```python
from build123d import *

# Parameters (mm, degrees)
F0_W     = 42
F0_H     = 82
F1_DEPTH = 3
F2_W     = 42
F2_H     = 82
F2_W_2   = 35
F2_H_2   = 76
F3_DEPTH = 18
F4_W     = 12
F4_H     = 82
F5_DEPTH = 3
F7_DEPTH = 25
F8_DEPTH = 25
F9_R     = 3
F10_R    = 5


with BuildPart() as f1:
    # F0 (on Top) → F1 (new body)
    with BuildSketch(Plane.XY):
        Rectangle(F0_W, F0_H)
    extrude(amount=F1_DEPTH)

    # F2 (on face) → F3 (join)
    with BuildSketch(Plane.XY.offset(3)):
        Rectangle(F2_W, F2_H)
        Rectangle(F2_W_2, F2_H_2, mode=Mode.SUBTRACT)
    extrude(amount=F3_DEPTH)

    # F4 (on face) → F5 (join)
    with BuildSketch(Plane.XY.offset(21)):
        with Locations((-23.5, 0)):
            Rectangle(F4_W, F4_H)
        with Locations((23.5, 0)):
            Rectangle(F4_W, F4_H)
    extrude(amount=F5_DEPTH)

    # F6 (on face) → F7 (cut)
    with BuildSketch(Plane(origin=(0, 0, 0), x_dir=(1, 0, 0), z_dir=(0, 0, -1))):
        Polygon((13, 7.8317355365), (13, 33), (3.5048450809, 33), (-13, 33), (-13, 14.662142843), (-13, -41), (13, -41), align=None)
    extrude(amount=-F7_DEPTH, mode=Mode.SUBTRACT)

    # F8 (cut): faces of the model
    f8_faces = [f1.faces().sort_by_distance(p)[0] for p in [
        (15.25, 38, 12),
        (-15.25, 38, 12),
    ]]
    extrude(f8_faces, amount=-F8_DEPTH, mode=Mode.SUBTRACT)

    # F9
    f9_edges = [f1.edges().sort_by_distance(p)[0] for p in [
        (-21, 0, 0),
        (0, -41, 0),
        (21, 0, 0),
        (-13, 41, 1.5),
        (13, 41, 1.5),
    ]]
    fillet(f9_edges, radius=F9_R)

    # F10
    f10_edges = [f1.edges().sort_by_distance(p)[0] for p in [
        (29.5, -41, 22.5),
        (-29.5, -41, 22.5),
        (-29.5, 41, 22.5),
        (29.5, 41, 22.5),
    ]]
    fillet(f10_edges, radius=F10_R)


solid = f1.part
```
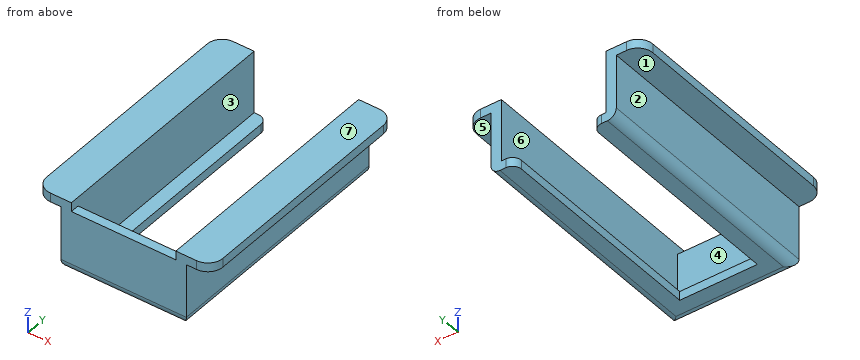
Check sheet for the modelled part. Datum: model origin and axes. Units: mm. Face numbers are marked on the shaded views. A direction names the side the tool comes from. Give positions to 0.01 mm unless a question says otherwise; leave off trailing zeros. Order: outer loops, then holes, each group sorted by start corner. A loop starts at its lowest first (then second) coordinate and runs counter-clockwise, first axis right, second up. Notation, with made-up numbers: (47, 32) -> (79, 32) arc R12 cw to (79, 55) -> close; hole circle Ø1 at (-15, 81.5). An arc over 180 degrees is marked (long way). Use CSV: the item, a comma, the result in double quotes. Start each with the question number.
1) Set-up check for the marked faces 5, 6 and 7: record each of +Z, -Z, +X, -X, +Y, -Y from which the full face is reachable in a straight line by a thin tool's end or side.
2) Mould release check, pull along X, two halves, no side actions. Record for the marked faces 1, 2, 3 and 4: released by +X, released by -X, zero draft, split by the parting line, or undercut.
3) Sectioned sample at D-D, the plane z = 5. Record the boundary of the cut face in (x, y), plus the area to 3 significant figures.
4) Sectioned sample at B-B, the plane x = 3. Record the boundary of the cut face in (y, z).
5) Sectioned sample at A-A, the plane z = 22.75. Record the boundary of the cut face in (x, y).
6) Sectioned sample at C-C, the plane y = -12.5. Record the boundary of the cut face in (x, z).
7) Material ranges on line 1 (X direction, y = 21.5, z = 14.75); line 2 (X direction, y = 2, z = 2.75); line 3 (Z direction, x = 22, y = 35), recorded low to high. Write a range as from..to.
8) Go/stop test with flat-tipped pins: P1, Ø2.5, axis at x = -1.5, z = 1.5, coming from the +Y side; P2, Ø2.5, axis at y = -5, z = 1, coming from the +X side; P3, Ø1.5, axis at x = -6.5, z = 16.5, coming from the +Y side. Record where each tip stops, or that it passes through.
Recorded:
1,face 5,"-Z, +X, +Y, -Y"
1,face 6,"+Z, +Y"
1,face 7,"+Z, +X, -X, +Y, -Y"
2,face 1,"zero draft"
2,face 2,"released by -X"
2,face 3,"undercut"
2,face 4,"undercut"
3,outline,"(-21, -41) -> (21, -41) -> (21, 41) -> (17.5, 41) -> (17.5, -38) -> (-17.5, -38) -> (-17.5, 41) -> (-21, 41) -> close"
3,area,"679 mm2"
4,outline,"(-41, 3) arc R3 ccw to (-38, 0) -> (-33, 0) -> (-33, 3) -> (-38, 3) -> (-38, 21) -> (-41, 21) -> close"
5,outline,"(-29.5, -36) arc R5 ccw to (-24.5, -41) -> (-17.5, -41) -> (-17.5, 41) -> (-24.5, 41) arc R5 ccw to (-29.5, 36) -> close; (17.5, -41) -> (24.5, -41) arc R5 ccw to (29.5, -36) -> (29.5, 36) arc R5 ccw to (24.5, 41) -> (17.5, 41) -> close"
6,outline,"(-29.5, 21) -> (-21, 21) -> (-21, 3) arc R3 ccw to (-18, 0) -> (-13, 0) -> (-13, 3) -> (-17.5, 3) -> (-17.5, 24) -> (-29.5, 24) -> close; (13, 0) -> (18, 0) arc R3 ccw to (21, 3) -> (21, 21) -> (29.5, 21) -> (29.5, 24) -> (17.5, 24) -> (17.5, 3) -> (13, 3) -> close"
7,line 1,"-21..-17.5, 17.5..21"
7,line 2,"-20.99..-13, 13..20.99"
7,line 3,"21..24"
8,P1,"y = -33"
8,P2,"x = 20.9"
8,P3,"y = -38"
